Geometry check sheet. Reference: drawing and pictorial views, mm from the part's lowest x, y, z. Give positions to 0.01 mm unless a question says otherwise; leave off trailing zeros. Order: outer loops, then holes, each group sorted by start corner. A loop starts at its lowest first (then second) coordinate and runs counter-clockwise, first axis right, second up. Notation, with made-up numbers: (-34, 67) - (7, 67) arc R28 ccw to (7, 93) - close; hole circle Ø2 at (42.25, 67.25). An arc over 180 degrees is marked (long way). Answer in a Markdown table with one row per item.
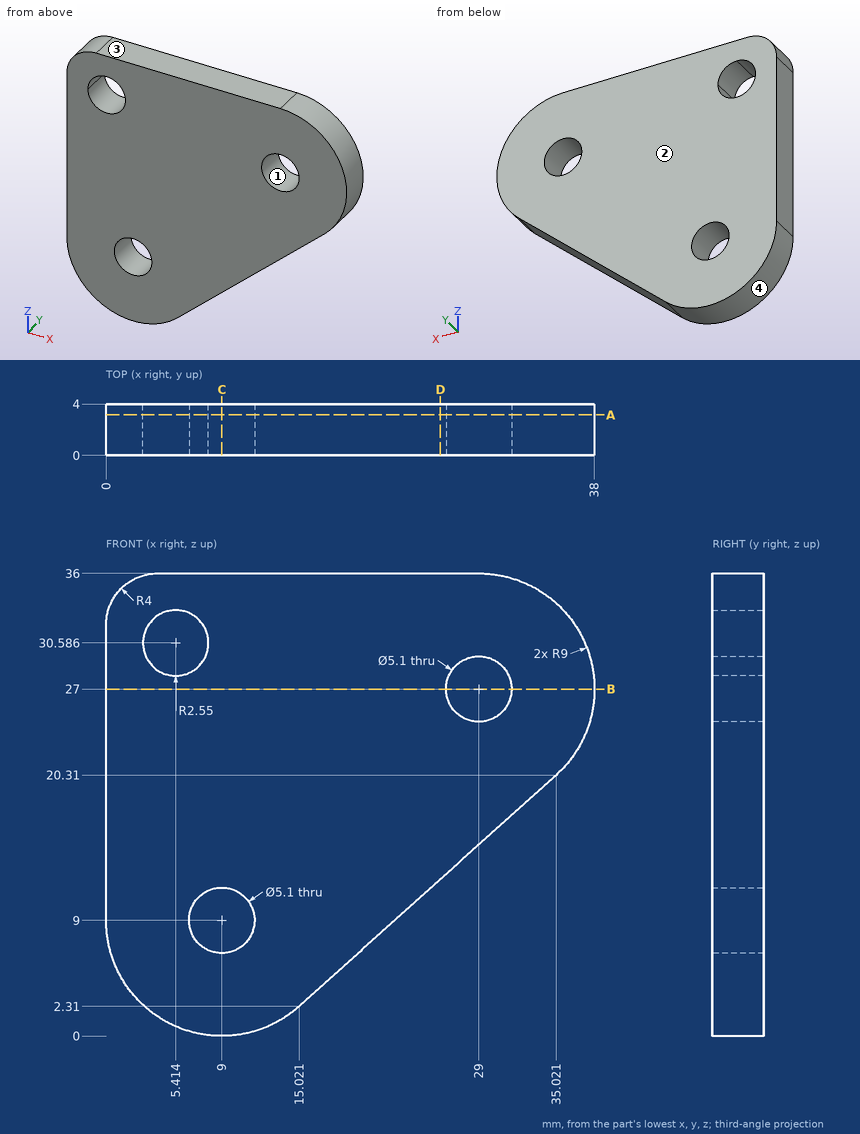
(1) Mould release check, pull along Z, two halves, no side actions. Record for the marked faces 1, 2, 3 and 4: pulls with the +Z half, pulls with the -Z half, needs draft (parallel to the pull), parting line crosses it, or undercut.
Geometry says:
| item | result |
|---|---|
| face 1 | undercut |
| face 2 | needs draft |
| face 3 | pulls with the +Z half |
| face 4 | pulls with the -Z half |
(2) Cross-section at A-A, the plane y = 3.15. Record the cut outline in (x, z), then the cut area to 3 significant figures.
Geometry says:
| item | result |
|---|---|
| outline | (0, 9) arc R9 ccw to (15.02, 2.31) - (35.02, 20.31) arc R9 ccw to (29, 36) - (4, 36) arc R4 ccw to (0, 32) - close; hole circle Ø5.1 at (5.41, 30.59); hole circle Ø5.1 at (9, 9); hole circle Ø5.1 at (29, 27) |
| area | 971 mm² |
(3) Cross-section at D-D, the plane x = 26. Record the cut outline in (y, z).
Geometry says:
| item | result |
|---|---|
| outline | (0, 12.19) - (4, 12.19) - (4, 36) - (0, 36) - close |
(4) Cross-section at B-B, the plane z = 27. Record the cut outline in (x, y), then the cut area to 3 significant figures.
Geometry says:
| item | result |
|---|---|
| outline | (0, 0) - (26.45, 0) - (26.45, 4) - (0, 4) - close; (31.55, 0) - (38, 0) - (38, 4) - (31.55, 4) - close |
| area | 132 mm² |
(5) Cross-section at C-C, the plane x = 9. Record the cut outline in (y, z), then the cut area to 3 significant figures.
Geometry says:
| item | result |
|---|---|
| outline | (0, 0) - (4, 0) - (4, 6.45) - (0, 6.45) - close; (0, 11.55) - (4, 11.55) - (4, 36) - (0, 36) - close |
| area | 124 mm² |
(6) Thickness scan on L1, parallel to X at y = 1.6, z = 27; L2, parallel to Z at x = 10, y = 2.8 (1 decimal); L3, parallel to Z at x = 11, y = 2 (1 decimal). Record the ranges inside material, lowest first.
Geometry says:
| item | result |
|---|---|
| L1 | 0 to 26.45, 31.55 to 38 |
| L2 | 0.1 to 6.7, 11.3 to 36 |
| L3 | 0.2 to 7.4, 10.6 to 36 |
(7) Gauge pin test, flat end, axial feed: P1, Ø8, axis at x = 9, z = 9, coming from the +Y side. Record the tip position at first contact, or that the pin passes through.
Geometry says:
| item | result |
|---|---|
| P1 | y = 4 |
